Source: CAD feature listing. Evaluate the final solid. Frame: model axes, mm. A direction names the side the tool comes from. Give positions to 0.01 mm unless a question says otherwise; leave off trailing zeros. Loops run counter-clockwise (first coordinate to the right, second up) from the corner with the lowest first, then second, coordinate; pieces in that order, holes last. Notation, with made-up numbers: (-13.5, -29) -> (29.5, -29) arc R15 cw to (29.5, 0) -> close; hole circle Ø2 at (77.25, -24.75). An arc over 180 degrees is marked (long way). Put each result on its own line as item: value.
```python
from build123d import *

# Parameters (mm, degrees)
EXTRUDE_1_DEPTH     = 320
SKETCH_2_R          = 1.5
CUT_EXTRUDE_1_DEPTH = 4


with BuildPart() as part:
    # Эскиз1 → Бобышка-Вытянуть1 (new body)
    with BuildSketch(Plane(origin=(0, 0, 0), x_dir=(0, 0, -1), z_dir=(1, 0, 0))):
        Polygon((0, 0), (-10, 0), (-10, 3), (-3, 3), (-3, 10), (0, 10), align=None)
    extrude(amount=EXTRUDE_1_DEPTH)

    # Эскиз2 → Вырез-Вытянуть1 (cut, through all)
    with BuildSketch(Plane.XY.offset(3)):
        with Locations((12.5, 6.5)):
            Circle(SKETCH_2_R)
        with Locations((307.5, 6.5)):
            Circle(SKETCH_2_R)
    extrude(amount=-CUT_EXTRUDE_1_DEPTH, mode=Mode.SUBTRACT)


solid = part.part
```
(1) Section A-A on y = 6.5. Return loops of the section in (x, z), then the cut area to 3 significant figures.
Calculated:
outline: (0, 0) -> (11, 0) -> (11, 3) -> (0, 3) -> close; (14, 0) -> (306, 0) -> (306, 3) -> (14, 3) -> close; (309, 0) -> (320, 0) -> (320, 3) -> (309, 3) -> close
area: 942 mm²
(2) Reachability of faces 1 (the flat face through (158, 6, 3)), 2 (the flat face through (158, 0, 5)) from +Z, -Z, +X, -X, +Y, -Y: full face, straight path, thin tool, end or side. Return the list, or none.
Calculated:
face 1: +Z, +X, -X, +Y
face 2: +Z, -Z, +X, -X, -Y
(3) First-contact query: P1, Ø2, axis at x = 133, y = 7.5, coming from the +Z side; P2, Ø4, axis at x = 242, z = 7.5, coming from the +Y side. Flat tips, straight axial feed; report the tip coordinate or a pass-through.
Calculated:
P1: stops at z = 3
P2: stops at y = 3
(4) Section B-B on z = 8.5. Return loops of the section in (x, y), then the cut area to 3 significant figures.
Calculated:
outline: (0, 0) -> (320, 0) -> (320, 3) -> (0, 3) -> close
area: 960 mm²
(5) Section C-C on x = 295. Return loops of the section in (y, z), then the cut area to 3 significant figures.
Calculated:
outline: (0, 0) -> (10, 0) -> (10, 3) -> (3, 3) -> (3, 10) -> (0, 10) -> close
area: 51.0 mm²
(6) Line query: probe 1 along Y at (x, z) = (12.5, 1.6); probe 2 along X at (y, z) = (5.5, 2.5); probe 3 along Z at (x, y) = (132, 7.5). Output: solid intervals per line, ascending. Write a range as from..to.
Calculated:
probe 1: y = 0..5, 8..10
probe 2: x = 0..11.38, 13.62..306.38, 308.62..320
probe 3: z = 0..3
